Build history of the part. All positions in model axes, mm. A direction names the side the tool comes from. Round coordinates to 2 decimals unless told otherwise and drop trailing zeros. Write each loop counter-clockwise with the first axis right and the second up, starting at its lowest first coordinate (ties: lowest second). Pieces come first, ordered by that corner, then holes. Notation, with made-up numbers: M 4.5,33.5 L 60.5,33.5 A21 cw 60.5,66.5 Z; hole C 84.25,61 d5. An arc over 180 degrees is marked long. Write item = value, one per line.
from build123d import *

# Parameters (mm, degrees)
F0_R     = 4.925
F1_DEPTH = 10
F2_DEPTH = 3


with BuildPart() as f1:
    # F0 (on Top) → F1 (new body)
    with BuildSketch(Plane.XY):
        with BuildLine():
            ThreePointArc((7.925, -25.425), (-1.326108, -17.611738), (-7.481199, -28.039821))
            ThreePointArc((-7.481199, -28.039821), (0, -33.35), (7.481199, -28.039821))
            ThreePointArc((7.481199, -28.039821), (7.813262, -26.751108), (7.925, -25.425))
        make_face()
        with Locations((0, -25.425)):
            Circle(F0_R, mode=Mode.SUBTRACT)
    extrude(amount=F1_DEPTH)

    # F0 (on Top) → F2 (join)
    with BuildSketch(Plane.XY):
        with BuildLine():
            Line((-6, 12.5), (-21.650635, 12.5))
            Line((-21.650635, 12.5), (-7.481199, -28.039821))
            ThreePointArc((-7.481199, -28.039821), (-1.326108, -17.611738), (7.925, -25.425))
            ThreePointArc((7.925, -25.425), (7.813262, -26.751108), (7.481199, -28.039821))
            Line((7.481199, -28.039821), (21.650635, 12.5))
            Line((21.650635, 12.5), (6, 12.5))
            Line((6, 12.5), (6, 0))
            ThreePointArc((6, 0), (0, -6), (-6, 0))
            Line((-6, 0), (-6, 12.5))
        make_face()
    extrude(amount=F2_DEPTH)


solid = f1.part
1. Band-saw the part on C-C (z = 7.75). List the corners of the cut face in (x, y) (3 decimals), plus the area to 3 significant figures.
Responses:
outline = M 7.481,-28.04 A7.925 ccw 7.925,-25.425 A7.925 ccw long Z; hole C 0,-25.425 d9.85
area = 121 mm²
2. Probe probe 1 along Y at (x, z) = (0, 2); probe 2 along Y at (x, z) = (0, 4.5); probe 3 along Z at (x, y) = (14, -7). List the from-to ranges inside material, lowest first.
Responses:
probe_1 = -33.35 to -30.35, -20.5 to -6
probe_2 = -33.35 to -30.35, -20.5 to -17.5
probe_3 = 0 to 3
3. Band-saw the part on D-D (y = -21.5). List the corners of the cut face in (x, z), plus the area to 3 significant figures.
Responses:
outline = M -9.77,0 L -2.97,0 L -2.97,10 L -6.88,10 L -6.88,3 L -9.77,3 Z; M 2.97,0 L 9.77,0 L 9.77,3 L 6.88,3 L 6.88,10 L 2.97,10 Z
area = 95.5 mm²
4. Flat gauge pins, fed straight in: pin 1 (0.9 mm diameter, centred on y = 4, z = 2, fed in from -X); pin 2 (10 mm diameter, centred on x = 1.5, y = 1.5, fed in from +Z); pin 3 (1 mm diameter, centred on y = -18.5, z = 4, fed in from +X). Where does each tip first touch, or does it go through?
Responses:
pin_1 = -18.84
pin_2 = 3
pin_3 = 4.64
5. Band-saw the part on A-A (y = -29). List the corners of the cut face in (x, z).
Responses:
outline = M -7.07,0 L -3.39,0 L -3.39,10 L -7.07,10 Z; M 3.39,0 L 7.07,0 L 7.07,10 L 3.39,10 Z
6. Band-saw the part on B-B (x = 0). List the corners of the cut face in (y, z).
Responses:
outline = M -33.35,0 L -30.35,0 L -30.35,10 L -33.35,10 Z; M -20.5,0 L -6,0 L -6,3 L -17.5,3 L -17.5,10 L -20.5,10 Z
7. Tool access for faces 5 (the face through (14, 12.5, 1)), 6 (the face through (6, 6, 1)): list every direction of +Z, -Z, +X, -X, +Y, -Y with a clear straight run to the whole face (end or side of a thin tool).
Responses:
face_5 = +Z, -Z, +X, -X, +Y
face_6 = +Z, -Z, +Y
8. Mould opens along X. For faces 1 (the face through (-4, -29, 10)), 2 (the face through (0, -6, 1)), 3 (the face through (-6, 6, 1)), 4 (the face through (14.47, -8.05, 1.48)) say: pulls with the +X half, pulls with the -X half, needs draft (parallel to the pull), parting line crosses it, or undercut.
Responses:
face_1 = needs draft
face_2 = undercut
face_3 = undercut
face_4 = pulls with the +X half
